from build123d import *

# Parameters (mm, degrees)
SKETCH_1_W                            = 40.5
SKETCH_1_H                            = 20
MG995_CASE_PHOTO_APPROX35_DEPTH       = 35
MOUNTING_EARS_APPROX54P5_START        = 25
SKETCH_2_W                            = 54.5
SKETCH_2_H                            = 20
MOUNTING_EARS_APPROX54P5_DEPTH        = 3
SKETCH_3_R                            = 9.5
RAISED_COVER_APPROX_DEPTH             = 38
SKETCH_4_R                            = 3
OUTPUT_SHAFT_ENVELOPE_NO_SPLINE_DEPTH = 42
EAR_HOLES_REFERENCE_47X10_DEPTH       = 58.18609971
EAR_HOLES_REFERENCE_47X10_DEPTH_BACK  = 58.18609971
SKETCH_5_R                            = 2


with BuildPart() as part:
    # 草图1 → MG995_case_photo_approx35 (new body)
    with BuildSketch(Plane.XY):
        with Locations((-10.25, 0)):
            Rectangle(SKETCH_1_W, SKETCH_1_H)
    extrude(amount=MG995_CASE_PHOTO_APPROX35_DEPTH)

    # 草图2 → Mounting_ears_APPROX54p5 (add)
    with BuildSketch(Plane.XY.offset(MOUNTING_EARS_APPROX54P5_START)):
        with Locations((-10.25, 0)):
            Rectangle(SKETCH_2_W, SKETCH_2_H)
    extrude(amount=MOUNTING_EARS_APPROX54P5_DEPTH)

    # 草图3 → Raised_cover_APPROX (add)
    with BuildSketch(Plane.XY):
        with Locations(Location((0, 0, 0), (0, 0, 180))):
            Circle(SKETCH_3_R)
    extrude(amount=RAISED_COVER_APPROX_DEPTH)

    # 草图4 → Output_shaft_envelope_NO_SPLINE (add)
    with BuildSketch(Plane.XY):
        with Locations(Location((0, 0, 0), (0, 0, 180))):
            Circle(SKETCH_4_R)
    extrude(amount=OUTPUT_SHAFT_ENVELOPE_NO_SPLINE_DEPTH)

    # 草图5 → Ear_holes_REFERENCE_47x10 (cut, two sides: drawn at the far end of the back side and taken through both)
    with BuildSketch(Plane.XY.offset(-EAR_HOLES_REFERENCE_47X10_DEPTH_BACK)):
        with Locations((-34, -5)):
            Circle(SKETCH_5_R)
        with Locations((-34, 5)):
            Circle(SKETCH_5_R)
        with Locations((13, -5)):
            Circle(SKETCH_5_R)
        with Locations((13, 5)):
            Circle(SKETCH_5_R)
    extrude(amount=EAR_HOLES_REFERENCE_47X10_DEPTH + EAR_HOLES_REFERENCE_47X10_DEPTH_BACK, mode=Mode.SUBTRACT)


solid = part.part
Verification items for the finished model (mm, model axes). A direction names the side the tool comes from. Coordinates: 2 decimals unless noted, no trailing zeros. Write each loop counter-clockwise with the first axis right and the second up, starting at its lowest first coordinate (ties: lowest second). Pieces come first, ordered by that corner, then holes. Notation, with made-up numbers: (2, 27) -> (31, 27) arc R13 ccw to (31, 49) -> close; hole circle Ø10 at (89, -37). An arc over 180 degrees is marked (long way). One line per item, written item: value. Start each with the question number.
Q1. Cross-section at B-B on y = 5. Enter the section's corners in (x, z).
Q2. Thickness scan on L1, parallel to Y at x = 13, z = 26.3; L2, parallel to X at y = 5, z = 27.2; L3, parallel to Z at x = -17, y = 9. Record the ranges inside material, lowest first. Write a range as from..to.
Q3. Access from +Z, -Z, +X, -X, +Y, -Y to the whole of each face (thin tool, end or side, straight path). Record for faces 1 (the flat face through (13, 0, 25)), 2 (the flat face through (13, 0, 28)), 3 (the flat face through (2.24, -2.24, 38)).
Q4. Cross-section at C-C on y = 0. Enter the section's corners in (x, z).
Q5. Cross-section at A-A on x = 13. Enter the section's corners in (y, z).
Q6. Mould release check, pull along Y, two halves, no side actions. Record for faces 4 (the cylindrical face through (2.059, 9.274, 36.479)), 5 (the cylindrical face through (-32.092, 5.601, 26.479)), 6 (the flat face through (-37.5, 0, 26)), 7 (the flat face through (-11, 10, 17)): pulls with the +Y half, pulls with the -Y half, needs draft (parallel to the pull), parting line crosses it, or undercut.
Q7. Go/stop test with flat-tipped pins: P1, Ø6, axis at y = 2.5, z = 16.5, coming from the -X side; P2, Ø6, axis at y = 7.5, z = 36.5, coming from the +X side; P3, Ø6.5, axis at x = -34, y = -5, coming from the -Z side. Record where each tip stops, or that it passes through.
Q8. Cross-section at D-D on x = 0. Enter the section's corners in (y, z).
Checked values:
1. outline: (-37.5, 25) -> (-36, 25) -> (-36, 28) -> (-37.5, 28) -> close; (-32, 25) -> (-30.5, 25) -> (-30.5, 0) -> (10, 0) -> (10, 25) -> (11, 25) -> (11, 28) -> (10, 28) -> (10, 35) -> (8.08, 35) -> (8.08, 38) -> (-8.08, 38) -> (-8.08, 35) -> (-30.5, 35) -> (-30.5, 28) -> (-32, 28) -> close; (15, 25) -> (17, 25) -> (17, 28) -> (15, 28) -> close
2. L1: y = -10..-7, -3..3, 7..10
2. L2: x = -37.5..-36, -32..11, 15..17
2. L3: z = 0..35
3. face 1: -Z, +X, +Y, -Y
3. face 2: +Z, +X, +Y, -Y
3. face 3: +Z
4. outline: (-37.5, 25) -> (-30.5, 25) -> (-30.5, 0) -> (10, 0) -> (10, 25) -> (17, 25) -> (17, 28) -> (10, 28) -> (10, 35) -> (9.5, 35) -> (9.5, 38) -> (3, 38) -> (3, 42) -> (-3, 42) -> (-3, 38) -> (-9.5, 38) -> (-9.5, 35) -> (-30.5, 35) -> (-30.5, 28) -> (-37.5, 28) -> close
5. outline: (-10, 25) -> (-7, 25) -> (-7, 28) -> (-10, 28) -> close; (-3, 25) -> (3, 25) -> (3, 28) -> (-3, 28) -> close; (7, 25) -> (10, 25) -> (10, 28) -> (7, 28) -> close
6. face 4: parting line crosses it
6. face 5: undercut
6. face 6: needs draft
6. face 7: pulls with the +Y half
7. P1: stops at x = -30.5
7. P2: stops at x = 10
7. P3: stops at z = 25
8. outline: (-10, 0) -> (10, 0) -> (10, 35) -> (9.5, 35) -> (9.5, 38) -> (3, 38) -> (3, 42) -> (-3, 42) -> (-3, 38) -> (-9.5, 38) -> (-9.5, 35) -> (-10, 35) -> close
